```python
from build123d import *

# Parameters (mm, degrees)
F0_R     = 14.351
F1_DEPTH = 7.9502
F2_R     = 15.748
F2_R_2   = 14.351
F3_DEPTH = 1.651
F4_DEPTH = 1.651
F5_DEPTH = 1.651
F6_DEPTH = 1.651


with BuildPart() as f1:
    # F0 (on Top) → F1 (new body)
    with BuildSketch(Plane.XY):
        with BuildLine():
            ThreePointArc((12.428331, 25.3365), (0, 18.161), (-12.428331, 25.3365))
            ThreePointArc((-12.428331, 25.3365), (-43.884105, 25.3365), (-28.156218, -1.905))
            ThreePointArc((-28.156218, -1.905), (-15.727887, -9.0805), (-15.727887, -23.4315))
            ThreePointArc((-15.727887, -23.4315), (0, -50.673), (15.727887, -23.4315))
            ThreePointArc((15.727887, -23.4315), (15.727887, -9.0805), (28.156218, -1.905))
            ThreePointArc((28.156218, -1.905), (43.884105, 25.3365), (12.428331, 25.3365))
        make_face()
        with Locations((0, -32.512)):
            Circle(F0_R, mode=Mode.SUBTRACT)
        Circle(F0_R, mode=Mode.SUBTRACT)
        with Locations((-28.156218, 16.256)):
            Circle(F0_R, mode=Mode.SUBTRACT)
        with Locations((28.156218, 16.256)):
            Circle(F0_R, mode=Mode.SUBTRACT)
    extrude(amount=F1_DEPTH)

    # F2 (on face) → F3 (cut)
    with BuildSketch(Plane.XY.offset(7.9502)):
        with Locations((-28.156218, 16.256)):
            Circle(F2_R)
        with Locations((-28.156218, 16.256)):
            Circle(F2_R_2, mode=Mode.SUBTRACT)
    extrude(amount=-F3_DEPTH, mode=Mode.SUBTRACT)

    # F2 (on face) → F4 (cut)
    with BuildSketch(Plane.XY.offset(7.9502)):
        with Locations((28.156218, 16.256)):
            Circle(F2_R)
        with Locations((28.156218, 16.256)):
            Circle(F2_R_2, mode=Mode.SUBTRACT)
    extrude(amount=-F4_DEPTH, mode=Mode.SUBTRACT)

    # F2 (on face) → F5 (cut)
    with BuildSketch(Plane.XY.offset(7.9502)):
        with Locations((0, -32.512)):
            Circle(F2_R)
        with Locations((0, -32.512)):
            Circle(F2_R_2, mode=Mode.SUBTRACT)
    extrude(amount=-F5_DEPTH, mode=Mode.SUBTRACT)

    # F2 (on face) → F6 (cut)
    with BuildSketch(Plane.XY.offset(7.9502)):
        Circle(F2_R)
        Circle(F2_R_2, mode=Mode.SUBTRACT)
    extrude(amount=-F6_DEPTH, mode=Mode.SUBTRACT)


solid = f1.part
```
Build history of the part. All positions in model axes, mm. A direction names the side the tool comes from. Round coordinates to 2 decimals unless told otherwise and drop trailing zeros. Loops run counter-clockwise (first coordinate to the right, second up) from the corner with the lowest first, then second, coordinate; pieces in that order, holes last.
Item 1: Saw through at B-B (y = -41). List the corners of the cut face in (x, z), then the cut area to 3 significant figures.
Item 2: Saw through at A-A (x = 0). List the corners of the cut face in (y, z), then the cut area to 3 significant figures.
Item 3: Which spindle directions (+Z, -Z, +X, -X, +Y, -Y) get a long thin tool onto all of the face, cutting with end or side? Do faces 4 (the face through (0.21, 18.163, 3.919)), 5 (the face through (12.423, 16.948, 7.136)). Say none if no direction does.
Item 4: Two-plate mould, pull along X, no slides. Class faces 1 (the face through (13.82, 16.89, 3.11)), 2 (the face through (-0.532, -50.665, 3.919)), 3 (the face through (-14, -8, 7.95)): released by +X, released by -X, zero draft, split by the parting line, or undercut.
Item 5: Saw through at D-D (z = 4.5). List the corners of the cut face in (x, y) (1 decimal), then the cut area to 3 significant figures.
Item 6: Drill centre lines: line 1 along Y through (x, z) = (-7, 7); line 2 along X through (y, z) = (25, 4.75); line 3 along X through (y, z) = (8.5, 1). Where is each one in solid material? Low to high.
Item 7: Saw through at C-C (x = 40.5). List the corners of the cut face in (y, z), then the cut area to 3 significant figures.
Item 8: Pin check, flat tips, straight feed: P1, Ø25, axis at x = 28.5, y = 14, coming from the +Z side; P2, Ø3, axis at x = 28, z = 6, coming from the +Y side; P3, Ø17, axis at x = 0, y = 0, coming from the -Z side; P4, Ø1.5, axis at x = -33.5, z = 3, coming from the -Y side. Stop position of each tip, or through.
Worked answers:
1. outline: (-16.06, 0) - (-11.57, 0) - (-11.57, 6.3) - (-13.26, 6.3) - (-13.26, 7.95) - (-16.06, 7.95) - close; (11.57, 0) - (16.06, 0) - (16.06, 7.95) - (13.26, 7.95) - (13.26, 6.3) - (11.57, 6.3) - close
1. area: 65.7 mm2
2. outline: (-50.67, 0) - (-46.86, 0) - (-46.86, 6.3) - (-48.26, 6.3) - (-48.26, 7.95) - (-50.67, 7.95) - close; (-18.16, 0) - (-14.35, 0) - (-14.35, 6.3) - (-15.75, 6.3) - (-15.75, 7.95) - (-16.76, 7.95) - (-16.76, 6.3) - (-18.16, 6.3) - close; (14.35, 0) - (18.16, 0) - (18.16, 7.95) - (15.75, 7.95) - (15.75, 6.3) - (14.35, 6.3) - close
2. area: 81.6 mm2
3. face 4: +Z, -Z, +Y
3. face 5: +Z
4. face 1: undercut
4. face 2: split by the parting line
4. face 3: zero draft
5. outline: (-28.2, -1.9) arc R14.4 cw to (-15.7, -23.4) arc R18.2 ccw (long way) to (15.7, -23.4) arc R14.4 cw to (28.2, -1.9) arc R18.2 ccw (long way) to (12.4, 25.3) arc R14.4 cw to (-12.4, 25.3) arc R18.2 ccw (long way) to start; hole circle Ø28.7 at (-28.2, 16.3); hole circle Ø28.7 at (0, -32.5); hole circle Ø28.7 at (0, 0); hole circle Ø28.7 at (28.2, 16.3)
5. area: 1,580 mm2
6. line 1: y = -49.27 to -46.62, -18.41 to -14.11, 14.11 to 19.98
6. line 2: x = -44.07 to -39.54, -16.78 to -12.23, 12.23 to 16.78, 39.54 to 44.07
6. line 3: x = -44.58 to -40.23, -16.08 to -11.56, 11.56 to 16.08, 40.23 to 44.58
7. outline: (2.93, 0) - (8.94, 0) - (8.94, 6.3) - (6.48, 6.3) - (6.48, 7.95) - (2.93, 7.95) - close; (23.58, 0) - (29.58, 0) - (29.58, 7.95) - (26.04, 7.95) - (26.04, 6.3) - (23.58, 6.3) - close
7. area: 87.3 mm2
8. P1: stops at z = 6.3
8. P2: stops at y = 34.42
8. P3: passes through
8. P4: stops at y = -1.31
